from build123d import *

# Parameters (mm, degrees)
SKICA1_R                 = 1.45
SKICA1_W                 = 4
SKICA1_H                 = 9.16588566
P_IDAT_VYSUNUT_M1_DEPTH  = 4
SKICA3_W                 = 4
SKICA3_H                 = 9.16588566
P_IDAT_VYSUNUT_M2_DEPTH  = 15
P_IDAT_VYSUNUT_M3_DEPTH  = 10
ODEBRAT_VYSUNUT_M2_DEPTH = 10
ODEBRAT_VYSUNUT_M3_DEPTH = 10
SKICA8_R                 = 2.75
ODEBRAT_VYSUNUT_M4_DEPTH = 10


with BuildPart() as part:
    # Skica1 → Přidat vysunutím1 (new body)
    # profile 1 of 2: a face of its own
    with BuildSketch(Plane.XY):
        Polygon((-7.778084737, -9.503012675), (-14.971883786, -9.503012675), (-14.971883786, -3.51452671), (11, 7.956888472), (11, -1.208997188), align=None)
        with Locations((-12.640965682, -7.067935851)):
            Circle(SKICA1_R, mode=Mode.SUBTRACT)
    # profile 2 of 2: a face of its own
    with BuildSketch(Plane.XY):
        with Locations((13, 3.373945642)):
            Rectangle(SKICA1_W, SKICA1_H)
    extrude(amount=P_IDAT_VYSUNUT_M1_DEPTH)

    # Skica3 → Přidat vysunutím2 (add, along a direction that is not the sketch's normal)
    with BuildSketch(Plane.XY.offset(4)):
        with Locations((13, 3.373945642)):
            Rectangle(SKICA3_W, SKICA3_H)
    extrude(amount=P_IDAT_VYSUNUT_M2_DEPTH, dir=(-0.5290758851456407, 0, 0.8485745151472301))

    # Skica5 → Přidat vysunutím3 (add)
    with BuildSketch(Plane(origin=(0, 7.956888472, 0), x_dir=(1, 0, 0), z_dir=(0, 1, 0))):
        Polygon((15, 0), (11, 0), (11, -4), (3.063861723, -16.728617727), (7.063861723, -16.728617727), (15, -4), align=None)
    extrude(amount=P_IDAT_VYSUNUT_M3_DEPTH)

    # Skica6 → Odebrat vysunutím2 (cut)
    with BuildSketch(Plane(origin=(9.716707036, 0, 6.058248609), x_dir=(-0.5290758851456409, 0, 0.8485745151472303), z_dir=(-0.8485745151472303, 0, -0.5290758851456409))):
        Polygon((-2.425536676, -1.208997188), (12.574463324, 10.009598213), (12.574463324, 17.956888472), (6.296672199, 17.956888472), (-7.12800363, 7.916488038), (-11.684978048, 8.945304904), (-10.179922277, 18.63037402), (-8.967516239, 18.63037402), (19.168665262, 18.63037402), (19.670350519, -6.557900971), (0.480889436, -6.557900971), align=None)
    extrude(amount=-ODEBRAT_VYSUNUT_M2_DEPTH, mode=Mode.SUBTRACT)

    # Skica7 → Odebrat vysunutím3 (cut)
    with BuildSketch(Plane(origin=(9.716707036, 0, 6.058248609), x_dir=(0.5290758851456409, 0, -0.8485745151472303), z_dir=(0.8485745151472303, 0, 0.5290758851456409))):
        Polygon((2.425536676, 17.956888472), (2.425536676, 11.433492981), (7.12800363, 7.916488038), (7.139324244, 7.919043865), (7.139324244, 17.956888472), align=None)
    extrude(amount=-ODEBRAT_VYSUNUT_M3_DEPTH, mode=Mode.SUBTRACT)

    # Skica8 → Odebrat vysunutím4 (cut)
    with BuildSketch(Plane(origin=(9.716707036, 0, 6.058248609), x_dir=(-0.5290758851456409, 0, 0.8485745151472303), z_dir=(-0.8485745151472303, 0, -0.5290758851456409))):
        with Locations((5.257931739, 11.090596363)):
            Circle(SKICA8_R)
    extrude(amount=-ODEBRAT_VYSUNUT_M4_DEPTH, mode=Mode.SUBTRACT)


solid = part.part
Could you check a few things on this model? Use its own coordinates, in mm. A direction names the side the tool comes from. Give positions to 0.01 mm unless a question says otherwise; leave off trailing zeros. Loops run counter-clockwise (first coordinate to the right, second up) from the corner with the lowest first, then second, coordinate; pieces in that order, holes last. Notation, with made-up numbers: (73.25, 79) -> (83.25, 79) arc R24 ccw to (83.25, 105) -> close; hole circle Ø6 at (-21.5, 32.5). An arc over 180 degrees is marked (long way). Answer as CSV lines item,"result". Start each with the question number.
(1) Which directions (+Z, -Z, +X, -X, +Y, -Y) give clear straight access to the entire face, cutting with the end or side of a thin tool? Please do faces 1 (the flat face through (-2, -3, 4)), 2 (the flat face through (8.51, 4.32, 11.16)), 3 (the flat face through (-2.17, 2.14, 1.97)), 4 (the flat face through (-11, -9.503, 2)), 5 (the flat face through (13, -1.209, 2)).
(2) If we section it at B-B on y = 2: Write out the boundary of the cut face in (x, z).
(3) If we section it at C-C on z = 4.75: Write out the boundary of the cut face in (x, y).
(4) I'm going to push flat-ended pins straight in: pin 1 Ø3 at (x, z) = (0.5, 5) entering from +Y; pin 2 Ø1.7 at (x, y) = (-12.64, -7.07) entering from +Z; pin 3 Ø2 at (x, y) = (-1.5, -4) entering from +Z; pin 4 Ø3 at (x, z) = (11, 8) entering from +Y. Where does each tip first touch, or does it pass through?
(5) If we section it at D-D on x = 11.75: Write out the boundary of the cut face in (y, z).
(6) We'd pull the mould along Z, two halves only. Please class faces 6 (the cylindrical face through (8.67, 8.406, 10.899)), 7 (the flat face through (0, 0, 0)), 8 (the flat face through (-14.972, -7, 2)), 9 (the flat face through (5, 13, 16.729)): released by +Z, released by -Z, zero draft, split by the parting line, or undercut.
(7) I need wall thicknesses on probe 1 along Z at (x, y) = (4.25, 0); probe 2 along X at (y, z) = (7.25, 9); probe 3 along Z at (x, y) = (10, 6). Which ranges of each line are inside material? Lowest first, please.
(8) If we section it at A-A on z = 1.5: Write out the boundary of the cut face in (x, y).
Computed:
1,face 1,"-X, +Y, -Y"
1,face 2,"+Z, -X, -Y"
1,face 3,"-Z, -X, +Y"
1,face 4,"+Z, -Z, +X, -X, -Y"
1,face 5,"+Z, -Z, +X, -Y"
2,outline,"(-2.49, 0) -> (15, 0) -> (15, 4) -> (11.61, 9.44) -> (8.73, 7.64) -> (11, 4) -> (-2.49, 4) -> close"
3,outline,"(10.53, -0.55) -> (12.2, -1.21) -> (14.53, -1.21) -> (14.53, 10.51) -> (10.53, 12.09) -> close"
4,pin 1,"stops at y = 3.81"
4,pin 2,"passes through"
4,pin 3,"stops at z = 4"
4,pin 4,"stops at y = 15.09"
5,outline,"(-1.21, 0) -> (8.6, 0) -> (14.44, 9.21) -> (1.8, 9.21) -> (-1.21, 4.47) -> close"
6,face 6,"undercut"
6,face 7,"released by -Z"
6,face 8,"zero draft"
6,face 9,"released by +Z"
7,probe 1,"z = 0 to 4"
7,probe 2,"x = 7.88 to 11.88"
7,probe 3,"z = 0 to 4, 5.6 to 12.02"
8,outline,"(-14.97, -9.5) -> (-7.78, -9.5) -> (11, -1.21) -> (15, -1.21) -> (15, 8.26) -> (11, 9.85) -> (11, 7.96) -> (-14.97, -3.51) -> close; hole circle Ø2.9 at (-12.64, -7.07)"
